Read the model definition and answer for the solid it produces. Units are mm, in the model's axes. Face numbers are marked on the shaded views. A direction names the side the tool comes from. Give positions to 0.01 mm unless a question says otherwise; leave off trailing zeros. Loops run counter-clockwise (first coordinate to the right, second up) from the corner with the lowest first, then second, coordinate; pieces in that order, holes last.
(1) Find section C-C, the plane x = 11. Write down the section's boundary in (y, z).
(2) Straight lines are drawn through the part: probe 1 along X at (y, z) = (7.75, -9.25); probe 2 along Y at (x, z) = (-8, 4.5) (3 decimals); probe 3 along Z at (x, y) = (4, -0.5). For each, find the intervals that lie inside material, in ascending order.
(3) Find section D-D, the plane z = -6.5. Write down the section's boundary in (x, y) (3 decimals).
(4) Each of these flat-tipped pins is pushed along its axis until it touches: P1, Ø14.5, axis at x = -7.5, z = 4, coming from the -Y side (3 decimals); P2, Ø12, axis at x = 55.5, z = 4.5, coming from the +Y side; P3, Ø14.5, axis at x = -7.5, z = 0, coming from the +Y side (3 decimals); P4, Ø6, axis at x = 24.5, z = -3, coming from the -Y side. Where does it stop, or does it pass through?
(5) Find section B-B, the plane y = 8. Write down the section's boundary in (x, z).
(6) Find section A-A, the plane y = 0. Write down the section's boundary in (x, z) (3 decimals), then the cut area to 3 significant figures.
(7) Determine the mould class of the marked faces 1, 2 and 3 for opening direction X: pulls with the +X half, pulls with the -X half, needs draft (parallel to the pull), parting line crosses it, or undercut.
(8) Which of the six approach directions +Z, -Z, +X, -X, +Y, -Y give full straight-line access (tool end or side, diameter ignored) to the marked faces 4, 5 and 6?
```python
from build123d import *

# Parameters (mm, degrees)
F0_R     = 3.175
F0_W     = 5.842
F0_H     = 12.7
F1_DEPTH = 3.175


with BuildPart() as f1:
    # F0 (on Front) → F1 (new body, symmetric)
    with BuildSketch(Plane.XZ):
        with BuildLine():
            Line((-0.9398, 0), (0, 0))
            Line((0, 0), (0, 12.7))
            Line((0, 12.7), (5.842, 12.7))
            Line((5.842, 12.7), (5.842, 15.24))
            Line((5.842, 15.24), (-0.508, 15.24))
            Line((-0.508, 15.24), (-10.88063, 3.847543))
            ThreePointArc((-10.88063, 3.847543), (-4.591961, 5.329721), (-0.9398, 0))
        make_face()
        with BuildLine():
            ThreePointArc((-8.182663, -5.506983), (-3.195791, -4.549339), (-0.9398, 0))
            ThreePointArc((-0.9398, 0), (-4.591961, 5.329721), (-10.88063, 3.847543))
            ThreePointArc((-10.88063, 3.847543), (-12.145978, -1.583727), (-8.182663, -5.506983))
        make_face()
        with Locations((-6.6548, 0)):
            Circle(F0_R, mode=Mode.SUBTRACT)
        with BuildLine():
            Line((5.842, 0), (0, 0))
            Line((0, 0), (-0.9398, 0))
            ThreePointArc((-0.9398, 0), (-3.195791, -4.549339), (-8.182663, -5.506983))
            Line((-8.182663, -5.506983), (5.842, -9.398))
            Line((5.842, -9.398), (5.842, 0))
        make_face()
        with Locations((2.921, 6.35)):
            Rectangle(F0_W, F0_H)
    extrude(amount=F1_DEPTH, both=True)

    # F0 (on Front) → F2 (revolve)
    with BuildSketch(Plane.XZ):
        Polygon((5.842, 12.7), (5.842, 0), (66.294, 0), (66.294, 12.7), (56.134, 12.7), (56.134, 10.16), (10.16, 10.16), (10.16, 12.7), align=None)
        with Locations((2.921, 6.35)):
            Rectangle(F0_W, F0_H)
    revolve(axis=Axis((33.147, 0, 0), (-1, 0, 0)))


solid = f1.part
```
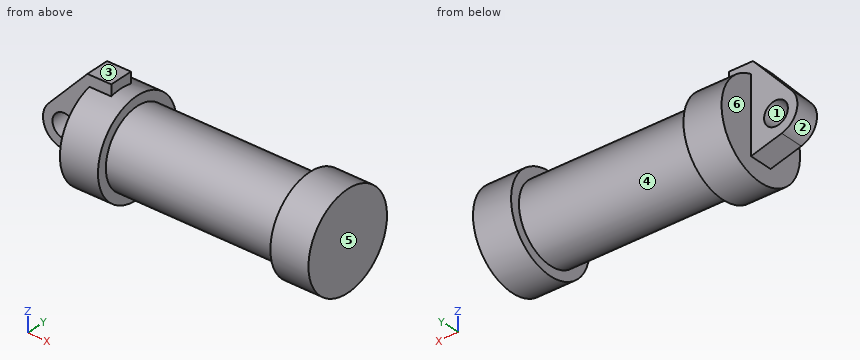
Entries:
1. outline: circle Ø20.32 at (0, 0)
2. probe 1: x = 0 to 10.16, 56.13 to 66.29
2. probe 2: y = -3.175 to 3.175
2. probe 3: z = -12.69 to 15.24
3. outline: (-4.603, -3.175) - (0, -3.175) - (0, -10.911) - (10.16, -10.911) - (10.16, -7.809) - (56.134, -7.809) - (56.134, -10.911) - (66.294, -10.911) - (66.294, 10.911) - (56.134, 10.911) - (56.134, 7.809) - (10.16, 7.809) - (10.16, 10.911) - (0, 10.911) - (0, 3.175) - (-4.603, 3.175) - close
4. P1: stops at y = -3.175
4. P2: stops at y = 12.7
4. P3: stops at y = 3.175
4. P4: stops at y = -10.16
5. outline: (0, -9.86) - (10.16, -9.86) - (10.16, -6.26) - (56.13, -6.26) - (56.13, -9.86) - (66.29, -9.86) - (66.29, 9.86) - (56.13, 9.86) - (56.13, 6.26) - (10.16, 6.26) - (10.16, 9.86) - (0, 9.86) - close
6. outline: (-10.881, 3.848) arc R5.715 ccw to (-8.183, -5.507) - (0, -7.777) - (0, -12.7) - (10.16, -12.7) - (10.16, -10.16) - (56.134, -10.16) - (56.134, -12.7) - (66.294, -12.7) - (66.294, 12.7) - (56.134, 12.7) - (56.134, 10.16) - (10.16, 10.16) - (10.16, 12.7) - (5.842, 12.7) - (5.842, 15.24) - (-0.508, 15.24) - close; hole circle Ø6.35 at (-6.655, 0)
6. area: 1,620 mm2
7. face 1: undercut
7. face 2: pulls with the -X half
7. face 3: needs draft
8. face 4: none
8. face 5: +Z, -Z, +X, +Y, -Y
8. face 6: -Z, -X
